```python
from build123d import *

# Parameters (mm, degrees)
SKETCH1_R           = 50
BOSS_EXTRUDE3_DEPTH = 2
SKETCH3_W           = 57
SKETCH3_H           = 77
SKETCH3_W_2         = 55
SKETCH3_H_2         = 75
BOSS_EXTRUDE4_DEPTH = 2
SKETCH4_W           = 84.733719196
SKETCH4_H           = 20.64189851
CUT_EXTRUDE1_DEPTH  = 2
SKETCH5_W           = 25.866082702
SKETCH5_H           = 94.035315438
CUT_EXTRUDE2_DEPTH  = 2
SKETCH6_R           = 1.5
CUT_EXTRUDE3_DEPTH  = 12
SKETCH7_R           = 1
CUT_EXTRUDE4_DEPTH  = 10.15


with BuildPart() as part:
    # Sketch1 → Boss-Extrude3 (new body)
    with BuildSketch(Plane(origin=(0, 0, 0), x_dir=(1, 0, 0), z_dir=(0, 1, 0))):
        with Locations(Location((0, 0, 0), (0, 0, 270))):
            Circle(SKETCH1_R)
    extrude(amount=BOSS_EXTRUDE3_DEPTH)

    # Sketch3 → Boss-Extrude4 (add)
    with BuildSketch(Plane(origin=(0, 2, 0), x_dir=(1, 0, 0), z_dir=(0, 1, 0))):
        Rectangle(SKETCH3_W, SKETCH3_H)
        Rectangle(SKETCH3_W_2, SKETCH3_H_2, mode=Mode.SUBTRACT)
    extrude(amount=BOSS_EXTRUDE4_DEPTH)

    # Sketch4 → Cut-Extrude1 (cut)
    with BuildSketch(Plane(origin=(0, 4, 0), x_dir=(1, 0, 0), z_dir=(0, 1, 0))):
        Rectangle(SKETCH4_W, SKETCH4_H)
    extrude(amount=-CUT_EXTRUDE1_DEPTH, mode=Mode.SUBTRACT)

    # Sketch5 → Cut-Extrude2 (cut)
    with BuildSketch(Plane(origin=(0, 4, 0), x_dir=(1, 0, 0), z_dir=(0, 1, 0))):
        Rectangle(SKETCH5_W, SKETCH5_H)
    extrude(amount=-CUT_EXTRUDE2_DEPTH, mode=Mode.SUBTRACT)

    # Sketch6 → Cut-Extrude3 (cut)
    with BuildSketch(Plane(origin=(0, 2, 0), x_dir=(1, 0, 0), z_dir=(0, 1, 0))):
        with Locations(Location((25, 22.2, 0), (0, 0, 270))):
            Circle(SKETCH6_R)
        with Locations(Location((-25, 22.2, 0), (0, 0, 270))):
            Circle(SKETCH6_R)
        with Locations(Location((9.8, -35, 0), (0, 0, 270))):
            Circle(SKETCH6_R)
        with Locations(Location((-9.8, -35, 0), (0, 0, 270))):
            Circle(SKETCH6_R)
    extrude(amount=-CUT_EXTRUDE3_DEPTH, mode=Mode.SUBTRACT)

    # Sketch7 → Cut-Extrude4 (cut)
    with BuildSketch(Plane(origin=(0, 2, 0), x_dir=(1, 0, 0), z_dir=(0, 1, 0))):
        with Locations(Location((-47.5, 0, 0), (0, 0, 270))):
            Circle(SKETCH7_R)
        with Locations(Location((47.5, 0, 0), (0, 0, 270))):
            Circle(SKETCH7_R)
    extrude(amount=-CUT_EXTRUDE4_DEPTH, mode=Mode.SUBTRACT)


solid = part.part
```
Can you work these out from the model? Positions are in its coordinate system, mm. Round coordinates to 2 decimals unless told otherwise and drop trailing zeros. Order: outer loops, then holes, each group sorted by start corner. A loop starts at its lowest first (then second) coordinate and runs counter-clockwise, first axis right, second up. Notation, with made-up numbers: (-11.75, 21) -> (40.25, 21) arc R22 cw to (40.25, 44) -> close; hole circle Ø4 at (19.5, 38.5). An arc over 180 degrees is marked (long way). Return JSON: item names as keys, results as strings. Group by question number.
1. If we section it at D-D, the plane z = 35: Write out the boundary of the cut face in (x, y), then the cut area to 3 significant figures.
2. We'd pull the mould along X, two halves only. Please class faces 1 (the face through (28, 4, 29)), 2 (the face through (8.9, 1, 33.8)), 3 (the face through (15.02, 0.99, 47.69)): released by +X, released by -X, zero draft, split by the parting line, or undercut.
3. If we section it at B-B, the plane x = 25: Write out the boundary of the cut face in (y, z).
4. Will these pins go through, and if not, where does the flat tip stop? pin 1 (2 mm diameter, centred on y = 2.5, z = 27.5, fed in from -X); pin 2 (1.6 mm diameter, centred on y = 2.5, z = -21.5, fed in from +X); pin 3 (2 mm diameter, centred on x = -20, y = 3.5, fed in from -Z).
5. I need wall thicknesses on line 1 (X direction, y = 1.65, z = 0); line 2 (X direction, y = 1.15, z = 35); line 3 (Z direction, x = 26.5, y = 2.6). Which ranges of each line are inside material? Lowest first, please. Write a range as [from, to].
6. If we section it at A-A, the plane y = 3: Write out the boundary of the cut face in (x, z), then the cut area to 3 significant figures.
7. If we section it at C-C, the plane z = -22.2: Write out the boundary of the cut face in (x, y).
Output values:
{
 "1": {"outline": "(-35.71, 0) -> (-11.3, 0) -> (-11.3, 2) -> (-27.5, 2) -> (-27.5, 4) -> (-28.5, 4) -> (-28.5, 2) -> (-35.71, 2) -> close; (-8.3, 0) -> (8.3, 0) -> (8.3, 2) -> (-8.3, 2) -> close; (11.3, 0) -> (35.71, 0) -> (35.71, 2) -> (28.5, 2) -> (28.5, 4) -> (27.5, 4) -> (27.5, 2) -> (11.3, 2) -> close", "area": "135 mm²"},
 "2": {"face 1": "zero draft", "face 2": "undercut", "face 3": "split by the parting line"},
 "3": {"outline": "(0, -43.3) -> (2, -43.3) -> (2, -38.5) -> (4, -38.5) -> (4, -37.5) -> (2, -37.5) -> (2, -23.7) -> (0, -23.7) -> close; (0, -20.7) -> (2, -20.7) -> (2, 37.5) -> (4, 37.5) -> (4, 38.5) -> (2, 38.5) -> (2, 43.3) -> (0, 43.3) -> close"},
 "4": {"pin 1": "x = -42.32", "pin 2": "x = 45.43", "pin 3": "z = -38.5"},
 "5": {"line 1": "[-50, -48.5], [-46.5, 46.5], [48.5, 50]", "line 2": "[-35.71, -11.3], [-8.3, 8.3], [11.3, 35.71]", "line 3": "[-38.5, -37.5], [37.5, 38.5]"},
 "6": {"outline": "(-28.5, -38.5) -> (-12.93, -38.5) -> (-12.93, -37.5) -> (-27.5, -37.5) -> (-27.5, -10.32) -> (-28.5, -10.32) -> close; (-28.5, 10.32) -> (-27.5, 10.32) -> (-27.5, 37.5) -> (-12.93, 37.5) -> (-12.93, 38.5) -> (-28.5, 38.5) -> close; (12.93, -38.5) -> (28.5, -38.5) -> (28.5, -10.32) -> (27.5, -10.32) -> (27.5, -37.5) -> (12.93, -37.5) -> close; (12.93, 37.5) -> (27.5, 37.5) -> (27.5, 10.32) -> (28.5, 10.32) -> (28.5, 38.5) -> (12.93, 38.5) -> close", "area": "171 mm²"},
 "7": {"outline": "(-44.8, 0) -> (-26.5, 0) -> (-26.5, 2) -> (-27.5, 2) -> (-27.5, 4) -> (-28.5, 4) -> (-28.5, 2) -> (-44.8, 2) -> close; (-23.5, 0) -> (23.5, 0) -> (23.5, 2) -> (-23.5, 2) -> close; (26.5, 0) -> (44.8, 0) -> (44.8, 2) -> (28.5, 2) -> (28.5, 4) -> (27.5, 4) -> (27.5, 2) -> (26.5, 2) -> close"}
}
